from build123d import *

# Parameters (mm, degrees)
CROQUIS1_W              = 25
CROQUIS1_H              = 25
SALIENTE_EXTRUIR1_DEPTH = 200
REDONDEO1_R             = 10
REDONDEO2_R             = 10
REDONDEO3_R             = 5
REDONDEO4_R             = 5
CROQUIS2_R              = 11
CROQUIS2_R_2            = 8.5
CORTAR_EXTRUIR1_DEPTH   = 6
CROQUIS3_R              = 8.5
CORTAR_EXTRUIR2_DEPTH   = 6
CROQUIS9_R              = 5.1
CROQUIS9_R_2            = 6
CORTAR_EXTRUIR6_DEPTH   = 30
CROQUIS13_W             = 1
CROQUIS13_H             = 5
CORTAR_EXTRUIR8_DEPTH   = 1
SALIENTE_EXTRUIR3_START = 3
CROQUIS14_R             = 11
CROQUIS14_R_2           = 5.1
SALIENTE_EXTRUIR3_DEPTH = 3
CROQUIS15_R             = 1.5
CORTAR_EXTRUIR9_DEPTH   = 16
CORTAR_EXTRUIR10_DEPTH  = 11
CORTAR_EXTRUIR12_REACH  = 205.101
CROQUIS18_W             = 1
CROQUIS18_H             = 1
CROQUIS20_W             = 17
CROQUIS20_H             = 100
CORTAR_EXTRUIR14_DEPTH  = 10
CROQUIS12_R             = 2.25
CORTAR_EXTRUIR7_DEPTH   = 204.100960116
CROQUIS21_W             = 58.914779702
CROQUIS21_H             = 35.760408196
CORTAR_EXTRUIR15_DEPTH  = 125
CROQUIS22_W             = 33.286593493
CROQUIS22_H             = 72.977677401
CORTAR_EXTRUIR16_DEPTH  = 8
REDONDEO5_R             = 10
CROQUIS24_R             = 8.5
CORTAR_EXTRUIR18_DEPTH  = 27
CROQUIS25_W             = 26.132042823
CROQUIS25_H             = 80
CORTAR_EXTRUIR19_DEPTH  = 5.5
REDONDEO6_R             = 10
REDONDEO7_R             = 10
CROQUIS27_W             = 27.934503923
CROQUIS27_H             = 80
CORTAR_EXTRUIR21_DEPTH  = 13.5
REDONDEO8_R             = 10
REDONDEO9_R             = 10


with BuildPart() as part:
    # Croquis1 → Saliente-Extruir1 (new body)
    with BuildSketch(Plane(origin=(0, 0, 0), x_dir=(1, 0, 0), z_dir=(0, 1, 0))):
        with Locations((12.5, 12.5)):
            Rectangle(CROQUIS1_W, CROQUIS1_H)
    extrude(amount=SALIENTE_EXTRUIR1_DEPTH)

    # Redondeo1
    redondeo1_edges = [part.edges().sort_by_distance(p)[0] for p in [
        (12.5, 0, -25),
    ]]
    fillet(redondeo1_edges, radius=REDONDEO1_R)

    # Redondeo2
    redondeo2_edges = [part.edges().sort_by_distance(p)[0] for p in [
        (12.5, 0, 0),
    ]]
    fillet(redondeo2_edges, radius=REDONDEO2_R)

    # Redondeo3
    redondeo3_edges = [part.edges().sort_by_distance(p)[0] for p in [
        (12.5, 200, 0),
    ]]
    fillet(redondeo3_edges, radius=REDONDEO3_R)

    # Redondeo4
    redondeo4_edges = [part.edges().sort_by_distance(p)[0] for p in [
        (12.5, 200, -25),
    ]]
    fillet(redondeo4_edges, radius=REDONDEO4_R)

    # Croquis2 → Cortar-Extruir1 (cut)
    with BuildSketch(Plane(origin=(25, 0, 0), x_dir=(0, 0, -1), z_dir=(1, 0, 0))):
        with Locations((12.5, 187.5)):
            Circle(CROQUIS2_R)
        with Locations(Location((12.5, 137.5, 0), (0, 0, 180))):
            Circle(CROQUIS2_R_2)
    extrude(amount=-CORTAR_EXTRUIR1_DEPTH, mode=Mode.SUBTRACT)

    # Croquis3 → Cortar-Extruir2 (cut)
    with BuildSketch(Plane.ZY):
        with Locations((-12.5, 12.5)):
            Circle(CROQUIS3_R)
        with Locations(Location((-12.5, 187.5, 0), (0, 0, 180))):
            Circle(CROQUIS3_R)
    extrude(amount=-CORTAR_EXTRUIR2_DEPTH, mode=Mode.SUBTRACT)

    # Croquis9 → Cortar-Extruir6 (cut)
    with BuildSketch(Plane(origin=(19, 0, 0), x_dir=(0, 0, -1), z_dir=(1, 0, 0))):
        with Locations((12.5, 187.5)):
            Circle(CROQUIS9_R)
        with Locations((12.5, 137.5)):
            Circle(CROQUIS9_R_2)
    extrude(amount=-CORTAR_EXTRUIR6_DEPTH, mode=Mode.SUBTRACT)

    # Croquis13 → Cortar-Extruir8 (cut)
    with BuildSketch(Plane(origin=(0, 0, -25), x_dir=(-1, 0, 0), z_dir=(0, 0, -1))):
        with Locations((-12.5, 187.04733642)):
            Rectangle(CROQUIS13_W, CROQUIS13_H)
    extrude(amount=-CORTAR_EXTRUIR8_DEPTH, mode=Mode.SUBTRACT)

    # Croquis14 → Saliente-Extruir3 (add)
    with BuildSketch(Plane(origin=(19, 0, 0), x_dir=(0, 0, -1), z_dir=(1, 0, 0)).offset(SALIENTE_EXTRUIR3_START)):
        with Locations((12.5, 187.5)):
            Circle(CROQUIS14_R)
        with Locations((12.5, 187.5)):
            Circle(CROQUIS14_R_2, mode=Mode.SUBTRACT)
    extrude(amount=-SALIENTE_EXTRUIR3_DEPTH)

    # Croquis15 → Cortar-Extruir9 (cut)
    with BuildSketch(Plane(origin=(22, 0, 0), x_dir=(0, 0, -1), z_dir=(1, 0, 0))):
        with Locations((17.980077554, 182.019922446)):
            Circle(CROQUIS15_R)
        with Locations((7.019922446, 182.019922446)):
            Circle(CROQUIS15_R)
        with Locations((7.019922446, 192.980077554)):
            Circle(CROQUIS15_R)
        with Locations((17.980077554, 192.980077554)):
            Circle(CROQUIS15_R)
    extrude(amount=-CORTAR_EXTRUIR9_DEPTH, mode=Mode.SUBTRACT)

    # Croquis16 → Cortar-Extruir10 (cut)
    with BuildSketch(Plane.ZY):
        Polygon((-14.829996635, 192.251844396), (-15.774368679, 195.344011075), (-18.924449599, 196.072244234), (-21.130158474, 193.708310713), (-20.185786429, 190.616144033), (-17.035705509, 189.887910875), align=None)
        Polygon((-17.251844396, 185.170003365), (-20.344011075, 184.225631321), (-21.072244234, 181.075550401), (-18.708310713, 178.869841526), (-15.616144033, 179.814213571), (-14.887910875, 182.964294491), align=None)
        Polygon((-7.748155604, 189.829996635), (-4.655988925, 190.774368679), (-3.927755766, 193.924449599), (-6.291689287, 196.130158474), (-9.383855967, 195.185786429), (-10.112089125, 192.035705509), align=None)
        Polygon((-10.170003365, 182.748155604), (-9.225631321, 179.655988925), (-6.075550401, 178.927755766), (-3.869841526, 181.291689287), (-4.814213571, 184.383855967), (-7.964294491, 185.112089125), align=None)
    extrude(amount=-CORTAR_EXTRUIR10_DEPTH, mode=Mode.SUBTRACT)

    # Cortar-Extruir12: up to this face of the body (flat: up to its plane)
    cortar_extruir12_end = Plane(part.part.faces().sort_by_distance((0, 98.930151157, -12.5))[0])
    # Croquis18 → Cortar-Extruir12 (cut, up to the picked face)
    with BuildSketch(Plane(origin=(25, 0, 0), x_dir=(0, 0, -1), z_dir=(1, 0, 0)), mode=Mode.PRIVATE) as cortar_extruir12_sk1:
        with Locations((24.5, 187.5)):
            Rectangle(CROQUIS18_W, CROQUIS18_H)
    cortar_extruir12_tool1 = split(extrude(cortar_extruir12_sk1.sketch, amount=-CORTAR_EXTRUIR12_REACH, mode=Mode.PRIVATE), bisect_by=cortar_extruir12_end, keep=Keep.BOTH, mode=Mode.PRIVATE)
    # Croquis18 → Cortar-Extruir12 (cut, up to the picked face)
    with BuildSketch(Plane(origin=(25, 0, 0), x_dir=(0, 0, -1), z_dir=(1, 0, 0)), mode=Mode.PRIVATE) as cortar_extruir12_sk2:
        with Locations((24.5, 137.5)):
            Rectangle(CROQUIS18_W, CROQUIS18_H)
    cortar_extruir12_tool2 = split(extrude(cortar_extruir12_sk2.sketch, amount=-CORTAR_EXTRUIR12_REACH, mode=Mode.PRIVATE), bisect_by=cortar_extruir12_end, keep=Keep.BOTH, mode=Mode.PRIVATE)
    add(cortar_extruir12_tool1.solids().sort_by(Axis((25, 187.5, -24.5), (-1, 0, 0)))[0], mode=Mode.SUBTRACT)
    add(cortar_extruir12_tool2.solids().sort_by(Axis((25, 137.5, -24.5), (-1, 0, 0)))[0], mode=Mode.SUBTRACT)

    # Croquis20 → Cortar-Extruir14 (cut)
    with BuildSketch(Plane.ZY):
        with Locations((-12.5, 75)):
            Rectangle(CROQUIS20_W, CROQUIS20_H)
    extrude(amount=-CORTAR_EXTRUIR14_DEPTH, mode=Mode.SUBTRACT)

    # Croquis12 → Cortar-Extruir7 (cut, through all)
    with BuildSketch(Plane(origin=(0, 0, -25), x_dir=(-1, 0, 0), z_dir=(0, 0, -1))):
        with Locations((-13.6, 187.5)):
            Circle(CROQUIS12_R)
    extrude(amount=-CORTAR_EXTRUIR7_DEPTH, mode=Mode.SUBTRACT)

    # Croquis21 → Cortar-Extruir15 (cut)
    with BuildSketch(Plane.XZ):
        with Locations((8.512503063, -10.548361389)):
            Rectangle(CROQUIS21_W, CROQUIS21_H)
    extrude(amount=-CORTAR_EXTRUIR15_DEPTH, mode=Mode.SUBTRACT)

    # Croquis22 → Cortar-Extruir16 (cut)
    with BuildSketch(Plane.ZY):
        with Locations((-13.640786543, 171.307251967)):
            Rectangle(CROQUIS22_W, CROQUIS22_H)
    extrude(amount=-CORTAR_EXTRUIR16_DEPTH, mode=Mode.SUBTRACT)

    # Redondeo5
    redondeo5_edges = [part.edges().sort_by_distance(p)[0] for p in [
        (12.5, 125, -25),
        (12.5, 125, 0),
    ]]
    fillet(redondeo5_edges, radius=REDONDEO5_R)

    # Croquis24 → Cortar-Extruir18 (cut)
    with BuildSketch(Plane(origin=(19, 0, 0), x_dir=(0, 0, -1), z_dir=(1, 0, 0))):
        with Locations(Location((12.5, 137.5, 0), (0, 0, 341.610158782))):
            Circle(CROQUIS24_R)
    extrude(amount=-CORTAR_EXTRUIR18_DEPTH, mode=Mode.SUBTRACT)

    # Croquis25 → Cortar-Extruir19 (cut)
    with BuildSketch(Plane(origin=(25, 0, 0), x_dir=(0, 0, -1), z_dir=(1, 0, 0))):
        with Locations((13.066021412, 135)):
            Rectangle(CROQUIS25_W, CROQUIS25_H)
    extrude(amount=-CORTAR_EXTRUIR19_DEPTH, mode=Mode.SUBTRACT)

    # Redondeo6
    redondeo6_edges = [part.edges().sort_by_distance(p)[0] for p in [
        (22.25, 175, -25),
    ]]
    fillet(redondeo6_edges, radius=REDONDEO6_R)

    # Redondeo7
    redondeo7_edges = [part.edges().sort_by_distance(p)[0] for p in [
        (22.25, 175, 0),
    ]]
    fillet(redondeo7_edges, radius=REDONDEO7_R)

    # Croquis27 → Cortar-Extruir21 (cut)
    with BuildSketch(Plane.ZY):
        with Locations((-13.967251962, 135)):
            Rectangle(CROQUIS27_W, CROQUIS27_H)
    extrude(amount=-CORTAR_EXTRUIR21_DEPTH, mode=Mode.SUBTRACT)

    # Redondeo8
    # the kernel refuses this fillet: 10 mm, written as the material it takes off along each edge
    with BuildSketch(Plane(origin=(38.5, 175, -25), x_dir=(0, 0, 1), z_dir=(-1, 0, 0))) as redondeo8_piece_1_section:
        with BuildLine():
            CenterArc((REDONDEO8_R, REDONDEO8_R), REDONDEO8_R, 180, 90)
            Line((0, REDONDEO8_R), (0, 0))
            Line((0, 0), (REDONDEO8_R, 0))
        make_face()
    redondeo8_piece_1 = extrude(amount=55.5, mode=Mode.PRIVATE)
    redondeo8_piece_1 = split(redondeo8_piece_1, bisect_by=Plane(origin=(19.5, 177.263951143, -22.736048857), z_dir=(1, 0, 0)), keep=Keep.TOP, mode=Mode.PRIVATE)
    add(redondeo8_piece_1, mode=Mode.SUBTRACT)
    with BuildSketch(Plane(origin=(13.5, 175, -25), x_dir=(0, 0, 1), z_dir=(-1, 0, 0))) as redondeo8_piece_2:
        with BuildLine():
            CenterArc((REDONDEO8_R, REDONDEO8_R), REDONDEO8_R, 180, 90)
            Line((0, REDONDEO8_R), (0, 0))
            Line((0, 0), (REDONDEO8_R, 0))
        make_face()
    extrude(amount=30.5, mode=Mode.SUBTRACT)

    # Redondeo9
    redondeo9_edges = [part.edges().sort_by_distance(p)[0] for p in [
        (10.75, 175, 0),
    ]]
    fillet(redondeo9_edges, radius=REDONDEO9_R)


solid = part.part
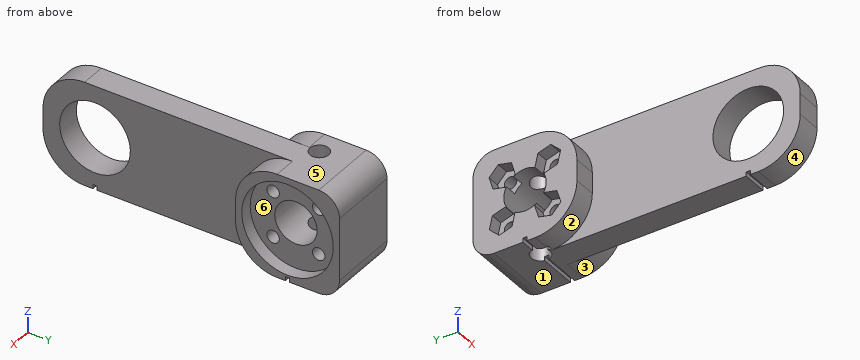
The listing builds one solid part. Answer for the finished solid, in the listing's coordinates (mm). Face numbers are marked on the shaded views. A direction names the side the tool comes from. Give positions to 0.01 mm unless a question says otherwise; leave off trailing zeros. Order: outer loops, then holes, each group sorted by start corner. A loop starts at its lowest first (then second) coordinate and runs counter-clockwise, first axis right, second up. Notation, with made-up numbers: (68, 60) - (74, 60) arc R22 ccw to (74, 66) - close; hole circle Ø8 at (38, 32.25). An arc over 180 degrees is marked (long way). Use one line per item in the form item = value.
1) The mould has two halves that part along Z. Classify the marked faces 4, 5 and 6: released by +Z, released by -Z, zero draft, split by the parting line, or undercut.
Verdict:
face_4 = released by -Z
face_5 = released by +Z
face_6 = undercut
2) Consider probe 1 along Y at (x, z) = (15.5, -12.5); probe 2 along X at (y, z) = (187, -18.25); probe 3 along Y at (x, z) = (12.5, -18). Determine where each line is inside the solid, lowest interval first. Write a range as [from, to].
Verdict:
probe_1 = [125, 129], [146, 182.4], [192.6, 200]
probe_2 = [8, 11.41], [15.79, 22]
probe_3 = [175.46, 180.52], [183.52, 185.54], [189.46, 191.48], [194.48, 200]
3) For the marked faces 1, 2 and 3, determine the directions among +Z, -Z, +X, -X, +Y, -Y from which every point of the face is accessible in a straight line to the end or side of a thin tool.
Verdict:
face_1 = -Z, +X, -X, +Y, -Y
face_2 = -Z, -X, -Y
face_3 = -Z, +X, -Y
4) Each of these flat-tipped pins is pushed along its axis until it touches: pin 1 (0.8 mm diameter, centred on x = 16, y = 137.5, fed in from -Z); pin 2 (5 mm diameter, centred on x = 13.6, y = 187.5, fed in from +Z); pin 3 (1.1 mm diameter, centred on x = 19.5, z = -24.5, fed in from +Y); pin 4 (8 mm diameter, centred on y = 168, z = -4.5, fed in from +X). Where does it stop, or does it pass through?
Verdict:
pin_1 = -24
pin_2 = 0
pin_3 = 198.07
pin_4 = 19.5
5) Find section D-D on y = 148.5. Determine the outline of the cut face in (x, z).
Verdict:
outline = (13.5, -25) - (19.5, -25) - (19.5, 0) - (13.5, 0) - close
6) Find section B-B on y = 139.5. Determine the outline of the cut face in (x, z), and give its area (3 significant figures).
Verdict:
outline = (13.5, -25) - (19.5, -25) - (19.5, -20.76) - (13.5, -20.76) - close; (13.5, -4.24) - (19.5, -4.24) - (19.5, 0) - (13.5, 0) - close
area = 50.9 mm^2
7) Find section C-C on x = 23.5. Determine the outline of the cut face in (y, z), and give its area (3 significant figures).
Verdict:
outline = (175, -15) arc R10 ccw to (185, -25) - (187, -25) - (187, -24) - (188, -24) - (188, -25) - (195, -25) arc R5 ccw to (200, -20) - (200, -5) arc R5 ccw to (195, 0) - (185, 0) arc R10 ccw to (175, -10) - close; hole circle Ø22 at (187.5, -12.5)
area = 190 mm^2
